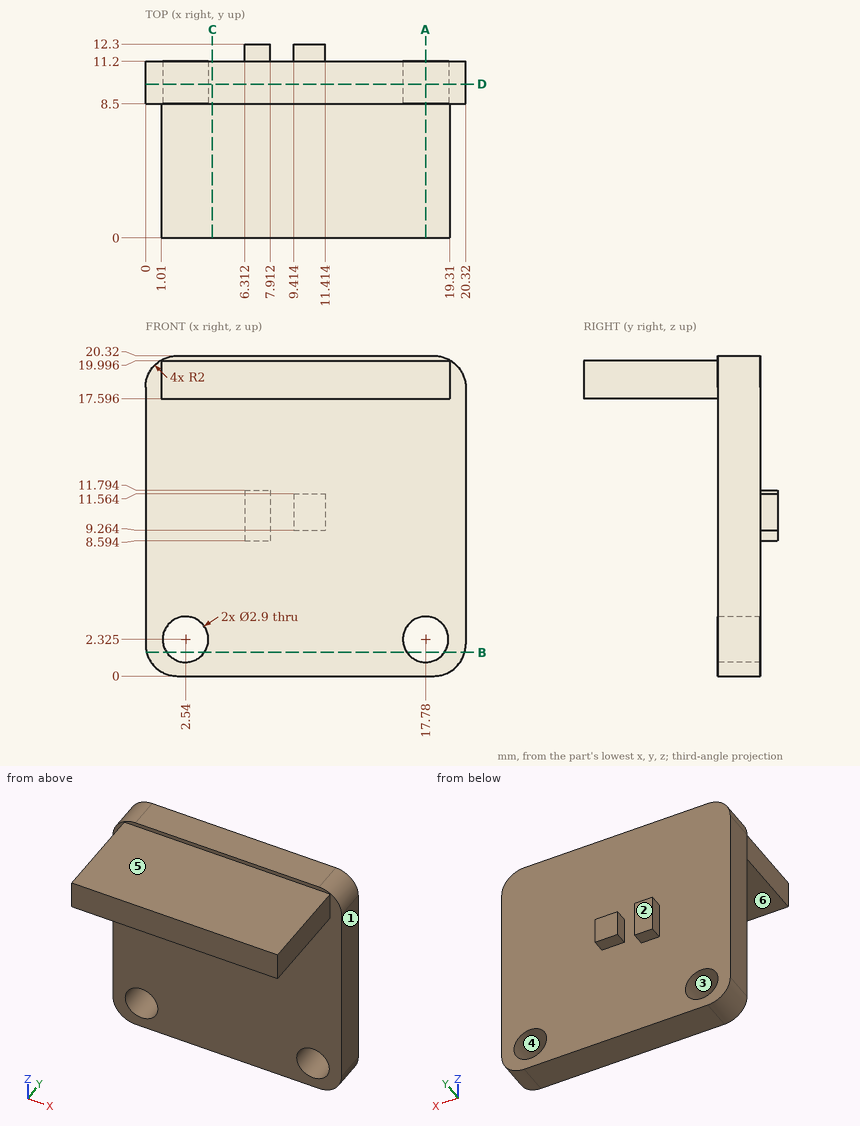
Check sheet for the drawn part. Datum: minimum x, y, z corner. Units: mm. A direction names the side the tool comes from. Coordinates: 2 decimals unless noted, no trailing zeros. Loops run counter-clockwise (first coordinate to the right, second up) from the corner with the lowest first, then second, coordinate; pieces in that order, holes last. Notation, with made-up numbers: (39, 58.25) -> (69, 58.25) arc R9 ccw to (69, 69.25) -> close; hole circle Ø9 at (51.25, 11.25). An arc over 180 degrees is marked (long way). Answer in a Markdown table with one row per item.
1) Section check B-B (z = 1.5). Record the cut outline in (x, y).
The answers:
| item | result |
|---|---|
| outline | (0.06, 8.5) -> (1.35, 8.5) -> (1.35, 11.2) -> (0.06, 11.2) -> close; (3.73, 8.5) -> (16.59, 8.5) -> (16.59, 11.2) -> (3.73, 11.2) -> close; (18.97, 8.5) -> (20.26, 8.5) -> (20.26, 11.2) -> (18.97, 11.2) -> close |
2) Section check D-D (y = 9.75). Record the cut outline in (x, z) (3 decimals).
The answers:
| item | result |
|---|---|
| outline | (0, 2) arc R2 ccw to (2, 0) -> (18.32, 0) arc R2 ccw to (20.32, 2) -> (20.32, 18.32) arc R2 ccw to (18.32, 20.32) -> (2, 20.32) arc R2 ccw to (0, 18.32) -> close; hole circle Ø2.9 at (2.54, 2.325); hole circle Ø2.9 at (17.78, 2.325) |
3) Access from +Z, -Z, +X, -X, +Y, -Y to the whole of each face (thin tool, end or side, straight path). Record for the marked faces 4, 5 and 6.
The answers:
| item | result |
|---|---|
| face 4 | +Y, -Y |
| face 5 | +Z, +X, -X, -Y |
| face 6 | -Z, +X, -X, -Y |
4) Scan lines: line 1 along X through (y, z) = (11.25, 9.5); line 2 along Y through (x, z) = (14.25, 13.25); line 3 along Y through (x, z) = (2, 19). Record each from-to range of solid material in increasing order. Write a range as from..to.
The answers:
| item | result |
|---|---|
| line 1 | x = 6.31..7.91, 9.41..11.41 |
| line 2 | y = 8.5..11.2 |
| line 3 | y = 0..11.2 |
5) Depth check by flat-ended pin: P1, Ø2.5, axis at y = 3, z = 19, coming from the -X side; P2, Ø2, axis at x = 2.5, y = 1, coming from the +Z side; P3, Ø12, axis at x = 15.5, z = 4, coming from the -Y side. Enter the tip coordinate at first touch or a pass-through.
The answers:
| item | result |
|---|---|
| P1 | stops at x = 1.01 |
| P2 | stops at z = 20 |
| P3 | stops at y = 8.5 |
6) Section check C-C (x = 4.25). Record the cut outline in (y, z).
The answers:
| item | result |
|---|---|
| outline | (0, 17.6) -> (8.5, 17.6) -> (8.5, 0) -> (11.2, 0) -> (11.2, 20.32) -> (8.5, 20.32) -> (8.5, 20) -> (0, 20) -> close |
7) Section check A-A (x = 17.78). Record the cut outline in (y, z) (3 decimals).
The answers:
| item | result |
|---|---|
| outline | (0, 17.596) -> (8.5, 17.596) -> (8.5, 3.775) -> (11.2, 3.775) -> (11.2, 20.32) -> (8.5, 20.32) -> (8.5, 19.996) -> (0, 19.996) -> close; (8.5, 0) -> (11.2, 0) -> (11.2, 0.875) -> (8.5, 0.875) -> close |
8) Draft check along X on the marked faces 1, 2 and 3. Enter one of: released by +X, released by -X, zero draft, split by the parting line, or undercut.
The answers:
| item | result |
|---|---|
| face 1 | released by +X |
| face 2 | zero draft |
| face 3 | undercut |
